Autodesk Inventor part; units mm, degrees
ref_plane "YZ Plane" through (0, 0, 0) normal (1, 0, 0) x (0, 1, 0)
ref_plane "XZ Plane" through (0, 0, 0) normal (0, 1, 0) x (-1, 0, 0)
ref_plane "XY Plane" through (0, 0, 0) normal (0, 0, 1) x (1, 0, 0)
sketch "Skizze1" plane through (0, 0, 0) normal (0, 0, 1) x (1, 0, 0)
  line L0 (0, 0) -> (24.6, 0)
  line L1 (0, 0) -> (0, 4)
  line L2 (0, 4) -> (8.6, 4)
  line L3 (8.6, 4) -> (8.6, 3)
  line L4 (8.6, 3) -> (24.6, 3)
  line L5 (24.6, 3) -> (24.6, 0)
  dimension "d0" = 8
  dimension "d1" = 6
  dimension "d2" = 8.6
  dimension "d3" = 16
revolve "Umdrehung1" add sketch "Skizze1" angle 360 about axis through (0, 0, 0) along (1, 0, 0)
sketch "Skizze2" plane through (0, 0, 0) normal (-1, 0, 0) x (0, 0, 1)
  point P0 (0, 0)
hole "Bohrung1" at (0, 0, 0) direction (1, 0, 0) diameter 3 end through all
hole "Bohrung2" at (0, 0, 0) direction (1, 0, 0) diameter 5 depth 4 tip angle 118
thread "Gewinde1"
chamfer "Fase1" distance 0.3 angle 45 2 edges at (24.6, -3, 0) (24.6, 0, -1.5)
properties part number "SlipRingExtender" material "Messing, weicher Gelbton"
Read the model definition and answer for the solid it produces. Units are mm, in the model's axes. A direction names the side the tool comes from. Give positions to 0.01 mm unless a question says otherwise; leave off trailing zeros. Order: outer loops, then holes, each group sorted by start corner. A loop starts at its lowest first (then second) coordinate and runs counter-clockwise, first axis right, second up.
(1) For a pull along Z with two mould halves and no side action, classify faces 4 (the cylindrical face through (14.59, -0.07, -1.5)), 5 (the flat face through (24.6, 2, -1)), 6 (the cylindrical face through (17, -3, 0)) as released by +Z, released by -Z, zero draft, split by the parting line, or undercut.
(2) Find section D-D (x = 14.5). Give the vertices of the cut face in (y, z), plus the area to 3 significant figures.
(3) For faces 1 (the cylindrical face through (4.36, -0.867, -3.905)), 2 (the cylindrical face through (2.03, 2.44, -0.54)), 3 (the flat face through (8.6, 1, 3)), determine the directions among +Z, -Z, +X, -X, +Y, -Y from which every point of the face is accessible in a straight line to the end or side of a thin tool.
(4) Given pin 1 (3 mm diameter, centred on y = 2.5, z = -2, fed in from +X); pin 2 (3 mm diameter, centred on x = 16, z = 3, fed in from -Y); pin 3 (2 mm diameter, centred on x = 6.5, y = 2, fed in from +Z), each flat-ended and moving along its own axis, determine where each tip first touches the part or whether it passes through.
(5) Find section C-C (x = 6.75). Give the vertices of the cut face in (y, z).
(6) Find section A-A (y = 0). Give the vertices of the cut face in (x, z).
(7) Straight lines are drawn through the part: L1, parallel to Z at x = 20, y = 0; L2, parallel to X at y = -3, z = 1.25; L3, parallel to Y at x = 3.75, z = -0.75. For each, find the intervals that lie inside material, in ascending order.
Result sheet:
1. face 4: undercut
1. face 5: zero draft
1. face 6: split by the parting line
2. outline: circle Ø6 at (0, 0); hole circle Ø3 at (0, 0)
2. area: 21.2 mm2
3. face 1: +X, -X
3. face 2: -X
3. face 3: +X
4. pin 1: stops at x = 24.6
4. pin 2: stops at y = -2.6
4. pin 3: stops at z = 3.87
5. outline: circle Ø8 at (0, 0); hole circle Ø3 at (0, 0)
6. outline: (0, -4) - (8.6, -4) - (8.6, -3) - (24.3, -3) - (24.6, -2.7) - (24.6, -1.8) - (24.3, -1.5) - (4.6, -1.5) - (4, -2.5) - (0, -2.5) - close; (0, 2.5) - (4, 2.5) - (4.6, 1.5) - (24.3, 1.5) - (24.6, 1.8) - (24.6, 2.7) - (24.3, 3) - (8.6, 3) - (8.6, 4) - (0, 4) - close
7. L1: z = -3 to -1.5, 1.5 to 3
7. L2: x = 0 to 8.6
7. L3: y = -3.93 to -2.38, 2.38 to 3.93
